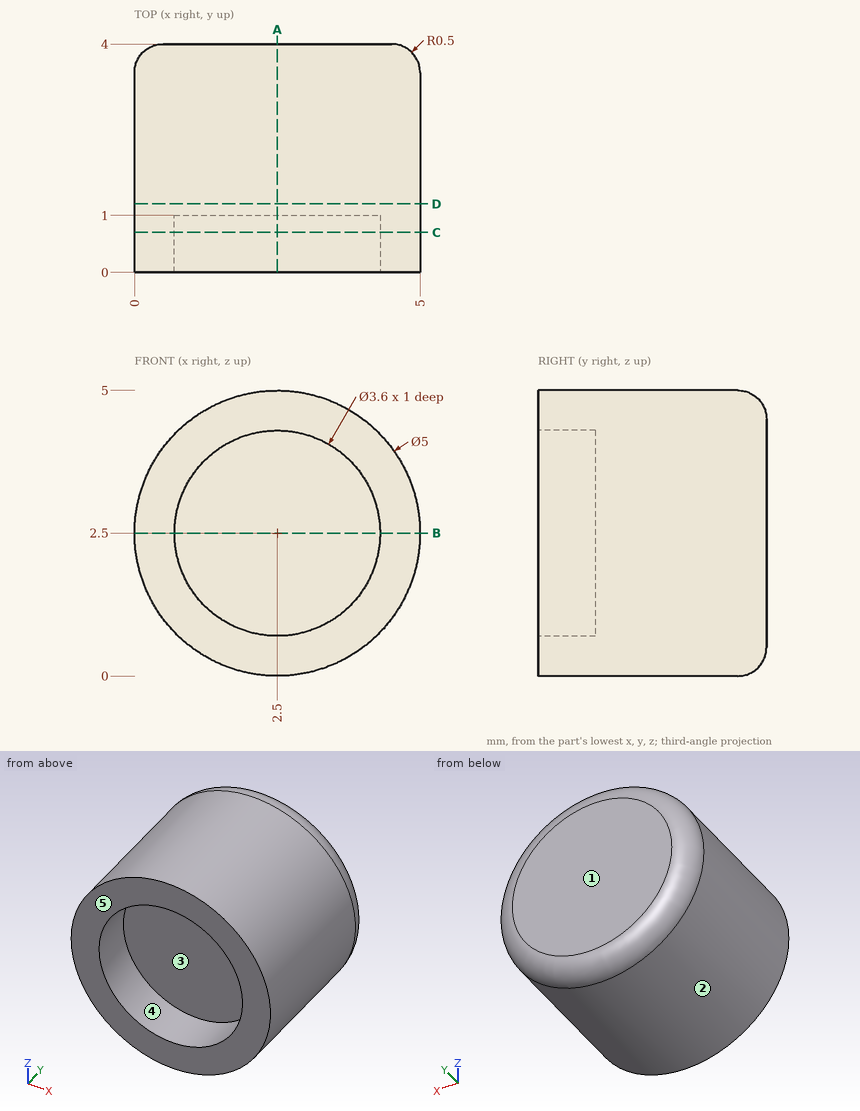
Design review of the part shown in the three views and the two pictorial views. Dimensions are in mm from the part's minimum x, y and z. A direction names the side the tool comes from. Round coordinates to 2 decimals unless told otherwise and drop trailing zeros. Write each loop counter-clockwise with the first axis right and the second up, starting at its lowest first coordinate (ties: lowest second). Pieces come first, ordered by that corner, then holes. Notation, with made-up numbers: (30, -1) -> (87, -1) arc R12 cw to (87, 16) -> close; hole circle Ø8 at (51, 19). An arc over 180 degrees is marked (long way). Write item = value, one per line. Start each with the question number.
1) Take a section at D-D, the plane y = 1.2. State the section outline as (x, z) points.
2) Clearance check with a flat-ended pin moving along its axis: pin 1 (1 mm diameter, centred on y = 1, z = 1.5, fed in from -X). State where the tip first meets the part, or that it passes through.
3) Take a section at B-B, the plane z = 2.5. State the section outline as (x, y) points, plus the area to 3 significant figures.
4) Take a section at A-A, the plane x = 2.5. State the section outline as (y, z) points, plus the area to 3 significant figures.
5) Wall thickness on probe 1 along Z at (x, y) = (2.5, 0.75); probe 2 along Y at (x, z) = (2.8, 0.85); probe 3 along X at (y, z) = (1.15, 3.5): over which ranges is each line inside the solid? List them lowest first. Write a range as from..to.
6) Mouldability with a two-part tool opening along X and no side actions: class the marked faces 1, 2 and 3 as +X half, -X half, draft (parallel to the pull), parting line (faces both ways), or undercut.
7) Tool access review of the marked faces 4 and 5: name each direction out of +Z, -Z, +X, -X, +Y, -Y from which nothing blocks a thin tool from reaching the whole face with its end or side.
8) Take a section at C-C, the plane y = 0.7. State the section outline as (x, z) points, plus the area to 3 significant figures.
Results list:
q1.outline = circle Ø5 at (2.5, 2.5)
q2.pin_1 = 0.05
q3.outline = (0, 0) -> (0.7, 0) -> (0.7, 1) -> (4.3, 1) -> (4.3, 0) -> (5, 0) -> (5, 3.5) arc R0.5 ccw to (4.5, 4) -> (0.5, 4) arc R0.5 ccw to (0, 3.5) -> close
q3.area = 16.3 mm²
q4.outline = (0, 0) -> (3.5, 0) arc R0.5 ccw to (4, 0.5) -> (4, 4.5) arc R0.5 ccw to (3.5, 5) -> (0, 5) -> (0, 4.3) -> (1, 4.3) -> (1, 0.7) -> (0, 0.7) -> close
q4.area = 16.3 mm²
q5.probe_1 = 0..0.7, 4.3..5
q5.probe_2 = 1..4
q5.probe_3 = 0.21..4.79
q6.face_1 = draft
q6.face_2 = parting line
q6.face_3 = undercut
q7.face_4 = -Y
q7.face_5 = +Z, -Z, +X, -X, -Y
q8.outline = circle Ø5 at (2.5, 2.5); hole circle Ø3.6 at (2.5, 2.5)
q8.area = 9.46 mm²
